from build123d import *

# Parameters (mm, degrees)
F1_DEPTH = 22
F2_DEPTH = 5
F3_DEPTH = 5
F4_DEPTH = 5
F5_R     = 10
F6_R     = 4.99999


# Not quite as in the source:
# - a fillet or chamfer is up to 0.001 mm smaller than in the source, because OpenCascade refuses the exact size


with BuildPart() as f1:
    # F0 (on Front) → F1 (new body)
    with BuildSketch(Plane.XZ):
        with BuildLine():
            Line((-80.1, 10.8671029838), (-80.1, -15.1328970162))
            Line((-80.1, -15.1328970162), (-80.1, -21.1328970162))
            ThreePointArc((-80.1, -21.1328970162), (-78.6355339059, -24.6684309221), (-75.1, -26.1328970162))
            Line((-75.1, -26.1328970162), (0, -26.1328970162))
            ThreePointArc((0, -26.1328970162), (-1.1715728753, -23.3044698915), (-4, -22.1328970162))
            Line((-4, -22.1328970162), (-69, -22.1328970162))
            ThreePointArc((-69, -22.1328970162), (-69.7071067812, -21.8400037974), (-70, -21.1328970162))
            Line((-70, -21.1328970162), (-70, -20.6328970162))
            ThreePointArc((-70, -20.6328970162), (-69.7071067812, -19.925790235), (-69, -19.6328970162))
            Line((-69, -19.6328970162), (6, -19.6328970162))
            ThreePointArc((6, -19.6328970162), (7.4142135624, -19.0471105786), (8, -17.6328970162))
            Line((8, -17.6328970162), (8, 10.8671029838))
            ThreePointArc((8, 10.8671029838), (7.4142135624, 12.2813165462), (6, 12.8671029838))
            Line((6, 12.8671029838), (4, 12.8671029838))
            Line((4, 12.8671029838), (0, 7.3002231531))
            Line((0, 7.3002231531), (2, 7.3002231531))
            ThreePointArc((2, 7.3002231531), (3.4142135624, 6.7144367155), (4, 5.3002231531))
            Line((4, 5.3002231531), (4, -13.6997768469))
            ThreePointArc((4, -13.6997768469), (3.4142135624, -15.1139904093), (2, -15.6997768469))
            Line((2, -15.6997768469), (-74.1, -15.6997768469))
            ThreePointArc((-74.1, -15.6997768469), (-75.5142135624, -15.1139904093), (-76.1, -13.6997768469))
            Line((-76.1, -13.6997768469), (-76.1, 5.3002231531))
            ThreePointArc((-76.1, 5.3002231531), (-75.5142135624, 6.7144367155), (-74.1, 7.3002231531))
            Line((-74.1, 7.3002231531), (-72.1, 7.3002231531))
            Line((-72.1, 7.3002231531), (-76.1, 12.8671029838))
            Line((-76.1, 12.8671029838), (-78.1, 12.8671029838))
            ThreePointArc((-78.1, 12.8671029838), (-79.5142135624, 12.2813165462), (-80.1, 10.8671029838))
        make_face()
    extrude(amount=F1_DEPTH)

    # F2 (add): a face of the model
    f2_faces = [f1.faces().sort_by_distance(p)[0] for p in [
        (-37.55, -11, -26.1328970162),
    ]]
    extrude(f2_faces, amount=F2_DEPTH)

    # F3 (add, through all): a face of the model
    f3_faces = [f1.faces().sort_by_distance(p)[0] for p in [
        (-75.1, -11, -28.6328970162),
    ]]
    extrude(f3_faces, amount=F3_DEPTH)

    # F4 (add): a face of the model
    f4_faces = [f1.faces().sort_by_distance(p)[0] for p in [
        (-77.6, -11, -26.1328970162),
    ]]
    extrude(f4_faces, amount=F4_DEPTH)

    # F5
    f5_edges = [f1.edges().sort_by_distance(p)[0] for p in [
        (-80.1, -11, -31.132897),
    ]]
    fillet(f5_edges, radius=F5_R)

    # F6 (radius 5 in the source; OpenCascade refuses exactly that, so slightly less here)
    f6_edges = [f1.edges().sort_by_distance(p)[0] for p in [
        (0, -11, -31.132897),
    ]]
    fillet(f6_edges, radius=F6_R)


solid = f1.part
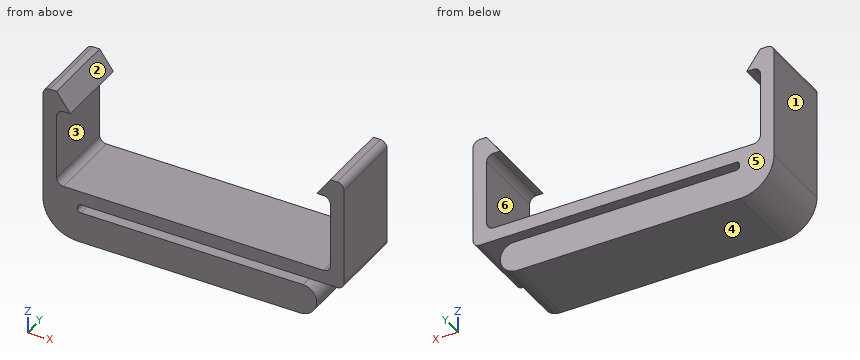
Geometry check sheet. Reference: the model listing, model coordinates, mm. Face numbers are marked on the shaded views. A direction names the side the tool comes from. Give positions to 0.01 mm unless a question says otherwise; leave off trailing zeros. Order: outer loops, then holes, each group sorted by start corner. A loop starts at its lowest first (then second) coordinate and runs counter-clockwise, first axis right, second up.
1) Cross-section at A-A (z = -9). Record the boundary of the cut face in (x, y).
Results are:
outline: (-80.1, -22) - (-76.1, -22) - (-76.1, 0) - (-80.1, 0) - close; (4, -22) - (8, -22) - (8, 0) - (4, 0) - close
2) Gauge pin test, flat ends, axial feed: pin 1 (2 mm diameter, centred on x = -73, y = -7, fed in from -Z); pin 2 (1 mm diameter, centred on y = -5.5, z = -24.5, fed in from -X); pin 3 (2 mm diameter, centred on x = 0.5, y = -8.5, fed in from -Z). Record the tip position at first contact, or that the pin passes through.
Results are:
pin 1: stops at z = -30.95
pin 2: stops at x = -79.68
pin 3: stops at z = -28.31
3) Material ranges on probe 1 along X at (y, z) = (-8.75, -1); probe 2 along Z at (x, y) = (-35, -11.75); probe 3 along Z at (x, y) = (-73.5, -1), recorded low to high.
Results are:
probe 1: x = -80.1 to -76.1, 4 to 8
probe 2: z = -31.13 to -22.13, -19.63 to -15.7
probe 3: z = -30.54 to -15.7, 7.3 to 9.25
4) Draft check along Z on the marked faces 4, 5 and 6. Enter one of: released by +Z, released by -Z, zero draft, split by the parting line, or undercut.
Results are:
face 4: released by -Z
face 5: zero draft
face 6: undercut
5) Cross-section at B-B (x = -55.5). Record the boundary of the cut face in (y, z).
Results are:
outline: (-22, -31.13) - (0, -31.13) - (0, -22.13) - (-22, -22.13) - close; (-22, -19.63) - (0, -19.63) - (0, -15.7) - (-22, -15.7) - close
6) Tool access check on the marked faces 1, 2 and 3. Record the directions out of +Z, -Z, +X, -X, +Y, -Y that give a thin tool (end or side, any length) a straight path to the whole face; none if there is none.
Results are:
face 1: +Z, -Z, -X, +Y, -Y
face 2: +Z, +Y, -Y
face 3: +Y, -Y
